```python
from build123d import *

# Parameters (mm, degrees)
SKETCH_1_W        = 12.8
SKETCH_1_H        = 7.3
SKETCH_1_R        = 1
EXTRUDE_1_DEPTH   = 3.2
SKETCH_2_W        = 0.5
SKETCH_2_H        = 3.2
EXTRUDE_1_2_DEPTH = 4
EXTRUDE_2_DEPTH   = 2


with BuildPart() as part:
    # Эскиз1 → Extrude 1 (new, symmetric)
    with BuildSketch(Plane.XY):
        with Locations((-6.4, 3.65)):
            Rectangle(SKETCH_1_W, SKETCH_1_H)
        with Locations((-9.65, 1.5)):
            Circle(SKETCH_1_R, mode=Mode.SUBTRACT)
        with Locations(Location((-3.15, 1.5, 0), (0, 0, 180))):
            Circle(SKETCH_1_R, mode=Mode.SUBTRACT)
    extrude(amount=EXTRUDE_1_DEPTH, both=True)

    # Эскиз2 → Extrude 1 2 (add)
    with BuildSketch(Plane.XZ):
        with Locations((-11.8, 0)):
            Rectangle(SKETCH_2_W, SKETCH_2_H)
        with Locations((-5.874787357, 0)):
            Rectangle(SKETCH_2_W, SKETCH_2_H)
        with Locations((-1, 0)):
            Rectangle(SKETCH_2_W, SKETCH_2_H)
    extrude(amount=EXTRUDE_1_2_DEPTH)

    # Эскиз3 → Вытянуть-Тонкостенный2 (add, symmetric)
    with BuildSketch(Plane.XY):
        with BuildLine():
            Line((-12.743673948, 7.056427884), (3.45, 10.801214984))
            Line((3.45, 10.801214984), (3.45, 11.461328502))
            ThreePointArc((3.45, 11.461328502), (3.861060305, 11.738598826), (4.25086812, 11.432168941))
            Line((4.25086812, 11.432168941), (4.732112122, 11.567831059))
            ThreePointArc((4.732112122, 11.567831059), (3.827123632, 12.23868926), (2.95, 11.531788258))
            Line((2.95, 11.531788258), (2.95, 11.198785016))
            Line((2.95, 11.198785016), (-12.856326052, 7.543572116))
            Line((-12.856326052, 7.543572116), (-12.743673948, 7.056427884))
        make_face()
    extrude(amount=EXTRUDE_2_DEPTH, both=True)


solid = part.part
```
Can you work these out from the model? Positions are in its coordinate system, mm. A direction names the side the tool comes from. Round coordinates to 2 decimals unless told otherwise and drop trailing zeros. Loops run counter-clockwise (first coordinate to the right, second up) from the corner with the lowest first, then second, coordinate; pieces in that order, holes last.
Item 1: Which directions (+Z, -Z, +X, -X, +Y, -Y) give clear straight access to the entire face, cutting with the end or side of a thin tool? Please do faces 4 (the flat face through (-5.625, -2, 0)), 5 (the flat face through (0, 4, 0)), 6 (the flat face through (-3.5, 9.4, 2)), 7 (the flat face through (-4.226, 9.026, 0.028)), 8 (the flat face through (-12.8, 4, 0)).
Item 2: If we mould it in two halves opening along X, with no side actions, what happens to faces 1 (the flat face through (-12.05, -2, 0)), 2 (the flat face through (-6, 4, -3.2)), 3 (the cylindrical face through (-2.36, 2.11, -0.04))? For each: +X half, -X half, draft (parallel to the pull), parting line (faces both ways), or undercut.
Item 3: Please list where these lines run through material, in increasing order: L1, parallel to X at y = -3, z = 0.25; L2, parallel to Y at x = -3.15, z = 0.5; L3, parallel to Y at x = -9.65, z = -0.75.
Item 4: Suppose I cut it at A-A, the plane y = 1.5. Write out the boundary of the cut face in (x, z).
Item 5: Suppose I cut it at D-D, the plane y = 10.25. Write out the boundary of the cut face in (x, z).
Item 6: Suppose I cut it at C-C, the plane x = -3.25. Write out the boundary of the cut face in (y, z).
Item 7: Will these pins go through, and if not, where does the flat tip stop? pin 1 Ø3 at (y, z) = (4, 0.5) entering from -X; pin 2 Ø0.6 at (x, y) = (-6, -1.5) entering from +Z; pin 3 Ø3.5 at (y, z) = (-1, -0.5) entering from +X.
Item 8: Suppose I cut it at B-B, the plane z = -0.75. Write out the boundary of the cut face in (x, y).
Reported:
1. face 4: +Z, -Z, -Y
1. face 5: +Z, -Z, +X, -Y
1. face 6: +Z, +X, -X, +Y
1. face 7: +Z, -Z, +X
1. face 8: +Z, -Z, -X, -Y
2. face 1: -X half
2. face 2: draft
2. face 3: undercut
3. L1: x = -12.05 to -11.55, -6.12 to -5.62, -1.25 to -0.75
3. L2: y = 0 to 0.5, 2.5 to 7.3, 9.27 to 9.79
3. L3: y = 0 to 0.5, 2.5 to 7.3, 7.77 to 8.29
4. outline: (-12.8, -3.2) - (-10.65, -3.2) - (-10.65, 3.2) - (-12.8, 3.2) - close; (-8.65, -3.2) - (-4.15, -3.2) - (-4.15, 3.2) - (-8.65, 3.2) - close; (-2.15, -3.2) - (0, -3.2) - (0, 3.2) - (-2.15, 3.2) - close
5. outline: (-1.15, -2) - (1.07, -2) - (1.07, 2) - (-1.15, 2) - close
6. outline: (0, -3.2) - (0.51, -3.2) - (0.51, 3.2) - (0, 3.2) - close; (2.49, -3.2) - (7.3, -3.2) - (7.3, 3.2) - (2.49, 3.2) - close; (9.25, -2) - (9.77, -2) - (9.77, 2) - (9.25, 2) - close
7. pin 1: stops at x = -12.8
7. pin 2: stops at z = 1.6
7. pin 3: stops at x = 0
8. outline: (-12.86, 7.54) - (-12.8, 7.3) - (-12.8, 0) - (-12.05, 0) - (-12.05, -4) - (-11.55, -4) - (-11.55, 0) - (-6.12, 0) - (-6.12, -4) - (-5.62, -4) - (-5.62, 0) - (-1.25, 0) - (-1.25, -4) - (-0.75, -4) - (-0.75, 0) - (0, 0) - (0, 7.3) - (-11.69, 7.3) - (3.45, 10.8) - (3.45, 11.46) arc R0.42 cw to (4.25, 11.43) - (4.73, 11.57) arc R0.92 ccw to (2.95, 11.53) - (2.95, 11.2) - close; hole circle Ø2 at (-9.65, 1.5); hole circle Ø2 at (-3.15, 1.5)
